CAD build for the part. Positions are in the model's coordinates, mm. Face numbers are marked on the shaded views. A direction names the side the tool comes from. Round coordinates to 2 decimals unless told otherwise and drop trailing zeros. Order: outer loops, then holes, each group sorted by start corner. A loop starts at its lowest first (then second) coordinate and runs counter-clockwise, first axis right, second up. Notation, with made-up numbers: M 82,69 L 105,69 A31 cw 105,96 Z; hole C 24.25,53 d3. An arc over 180 degrees is marked long. Answer as a JSON object with one key per item and string values.
```python
from build123d import *

# Parameters (mm, degrees)
F1_DEPTH = 25.4
F2_W     = 76.2
F2_H     = 12.7
F3_DEPTH = 12.7
F5_DEPTH = 12.7


with BuildPart() as f1:
    # F0 (on Top) → F1 (new body)
    with BuildSketch(Plane.XY):
        with BuildLine():
            Line((-95.25, 0), (0, 0))
            Line((0, 0), (0, 95.25))
            ThreePointArc((0, 95.25), (-67.351921, 67.351921), (-95.25, 0))
        make_face()
    extrude(amount=-F1_DEPTH)

    # F2 (on face) → F3 (cut)
    with BuildSketch(Plane.XZ):
        with Locations((-47.625, -12.7)):
            Rectangle(F2_W, F2_H)
    extrude(amount=-F3_DEPTH, mode=Mode.SUBTRACT)

    # F4 (on face) → F5 (join)
    with BuildSketch(Plane.YZ):
        Polygon((9.525, -6.35), (9.525, -12.7), (9.525, -19.05), (47.625, -19.05), (85.725, -19.05), (85.725, -12.7), (85.725, -6.35), (47.625, -6.35), align=None)
    extrude(amount=F5_DEPTH)


solid = f1.part
```
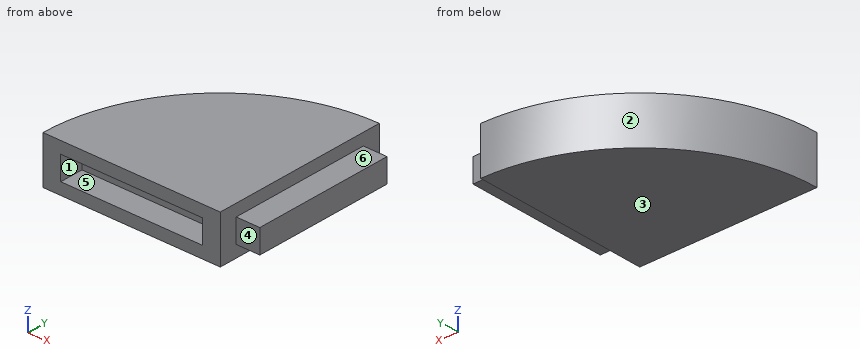
Item 1: 3-axis set-ups, long thin cutter, end or side, ignore diameter. For the marked faces 4, 5 and 6: which of +Z, -Z, +X, -X, +Y, -Y reach the whole face in a straight line?
Worked answers:
{"face 4": "+Z, -Z, +X, -Y", "face 5": "-Y", "face 6": "+Z, +X, +Y, -Y"}
Item 2: Saw through at B-B on y = 38.5. List the corners of the cut face in (x, z).
Worked answers:
{"outline": "M -87.12,-25.4 L 0,-25.4 L 0,-19.05 L 12.7,-19.05 L 12.7,-6.35 L 0,-6.35 L 0,0 L -87.12,0 Z"}
Item 3: Two-plate mould, pull along X, no slides. Class the marked faces 1, 2 and 3: released by +X, released by -X, zero draft, split by the parting line, or undercut.
Worked answers:
{"face 1": "undercut", "face 2": "released by -X", "face 3": "zero draft"}
Item 4: Saw through at C-C on z = -23.5. List the corners of the cut face in (x, y).
Worked answers:
{"outline": "M -95.25,0 L 0,0 L 0,95.25 A95.25 ccw Z"}
Item 5: Drop flat-ended pins along their axis: pin 1 Ø5 at (x, z) = (-53, -13) entering from -Y; pin 2 Ø6.5 at (x, z) = (8.5, -11.5) entering from -Y (3 decimals); pin 3 Ø3 at (x, z) = (-75, -5) entering from +Y. Give the stop position or say it passes through.
Worked answers:
{"pin 1": "stops at y = 12.7", "pin 2": "stops at y = 9.525", "pin 3": "stops at y = 60.58"}
Item 6: Saw through at D-D on x = 3. List the corners of the cut face in (y, z) (3 decimals).
Worked answers:
{"outline": "M 9.525,-19.05 L 85.725,-19.05 L 85.725,-6.35 L 9.525,-6.35 Z"}
Item 7: Wall check: line 1 along Z through (x, y) = (-67, 5.5); line 2 along X through (y, z) = (7.5, -9.75) (3 decimals); line 3 along Z through (x, y) = (6, 82). Give the ranges that are in metal, low to high. Write a range as [from, to].
Worked answers:
{"line 1": "z = [-25.4, -19.05], [-6.35, 0]", "line 2": "x = [-94.954, -85.725], [-9.525, 0]", "line 3": "z = [-19.05, -6.35]"}
Item 8: Saw through at A-A on x = -48. List the corners of the cut face in (y, z), and give its area (3 significant figures).
Worked answers:
{"outline": "M 0,-25.4 L 82.27,-25.4 L 82.27,0 L 0,0 L 0,-6.35 L 12.7,-6.35 L 12.7,-19.05 L 0,-19.05 Z", "area": "1,930 mm2"}
